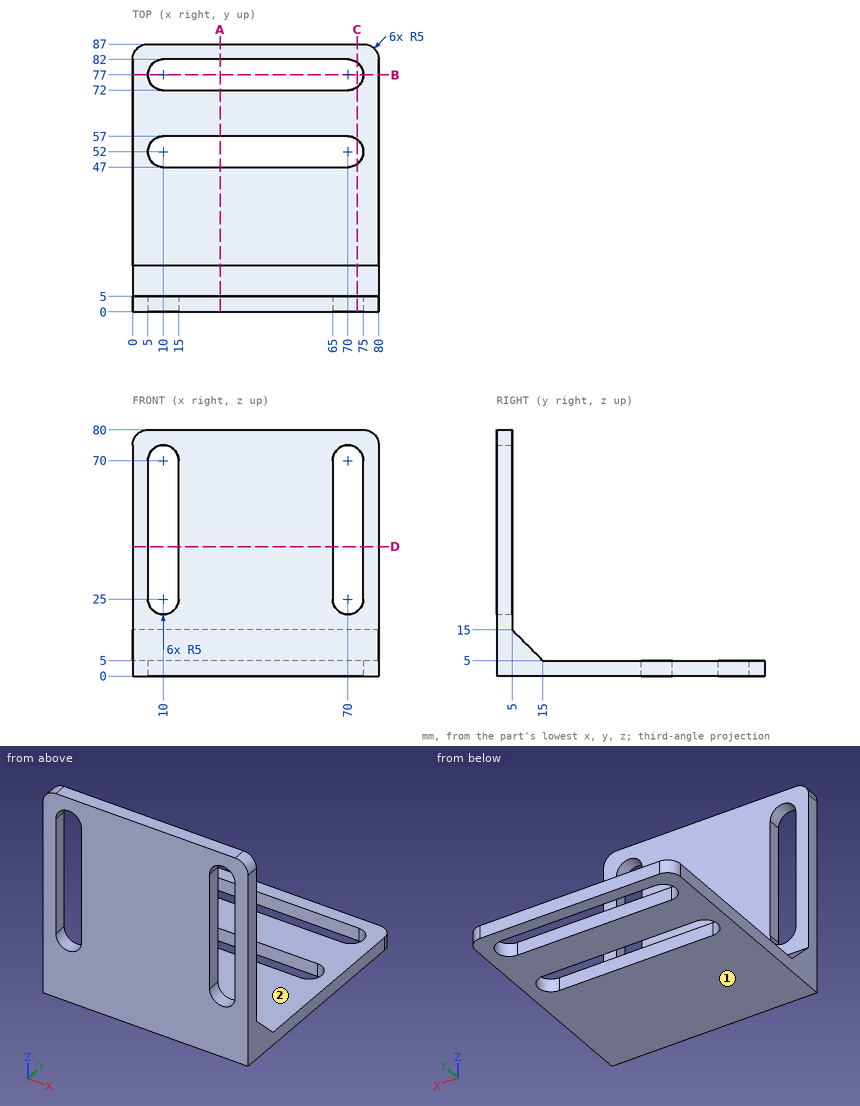
Here's the drawing with two shaded views (mm, measured from the low corner). I have some questions. A direction names the side the tool comes from. Round coordinates to 2 decimals unless told otherwise and drop trailing zeros. Write each loop counter-clockwise with the first axis right and the second up, starting at its lowest first coordinate (ties: lowest second). Pieces come first, ordered by that corner, then holes. Notation, with made-up numbers: M 85,-10 L 97,-10 A30 cw 97,17 Z; hole C -18.75,-13 d10. An arc over 180 degrees is marked long. Answer in a Markdown table with one row per item. Add a question column.
Q1. Will these pins go through, and if not, where does the flat tip stop? pin 1 Ø19.5 at (x, z) = (47.5, 57) entering from +Y; pin 2 Ø3 at (x, y) = (32.5, 57) entering from +Z.
Q2. Imagine slicing it at A-A (x = 28.5). Please give me the cut outline in (y, z), then the cut area to 3 significant figures.
Q3. Imagine slicing it at C-C (x = 73). Please give me the cut outline in (y, z).
Q4. Imagine slicing it at D-D (z = 42). Please give me the cut outline in (x, y), then the cut area to 3 significant figures.
Q5. If I drill on line 1 (Y direction, x = 32.5, z = 41.5); line 2 (Y direction, x = 77, z = 9), over which ranges is the centre line in solid material (lowest first)? Write a range as from..to.
Q6. On a 3-axis mill with a long thin cutter (end or side, diameter ignored), from which of +Z, -Z, +X, -X, +Y, -Y can I reach the whole of each face in a straight line? I mean the marked faces 1 and 2. Say none if no direction works.
Q7. Imagine slicing it at B-B (y = 77). Please give me the cut outline in (x, z), then the cut area to 3 significant figures.
Values:
| question | item | result |
|---|---|---|
| 1 | pin 1 | y = 5 |
| 1 | pin 2 | z = 5 |
| 2 | outline | M 0,0 L 47,0 L 47,5 L 15,5 L 5,15 L 5,80 L 0,80 Z; M 57,0 L 72,0 L 72,5 L 57,5 Z; M 82,0 L 87,0 L 87,5 L 82,5 Z |
| 2 | area | 760 mm^2 |
| 3 | outline | M 0,0 L 48,0 L 48,5 L 15,5 L 5,15 L 5,21 L 0,21 Z; M 0,74 L 5,74 L 5,80 L 0,80 Z; M 56,0 L 73,0 L 73,5 L 56,5 Z; M 81,0 L 87,0 L 87,5 L 81,5 Z |
| 4 | outline | M 0,0 L 5,0 L 5,5 L 0,5 Z; M 15,0 L 65,0 L 65,5 L 15,5 Z; M 75,0 L 80,0 L 80,5 L 75,5 Z |
| 4 | area | 300 mm^2 |
| 5 | line 1 | 0..5 |
| 5 | line 2 | 0..11 |
| 6 | face 1 | -Z, +X, -X, +Y, -Y |
| 6 | face 2 | +Z, +X, -X, +Y |
| 7 | outline | M 0,0 L 5,0 L 5,5 L 0,5 Z; M 75,0 L 80,0 L 80,5 L 75,5 Z |
| 7 | area | 50.0 mm^2 |
